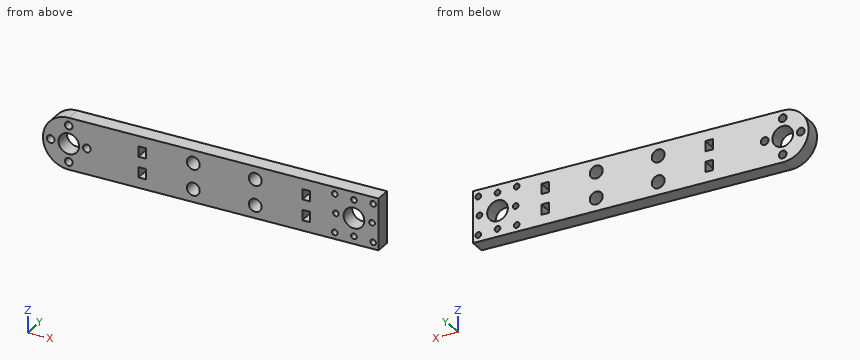
from build123d import *

# Parameters (mm, degrees)
EXTRUDE_1_DEPTH     = 6
SKETCH_2_R          = 1.5
SKETCH_2_R_2        = 4
CUT_EXTRUDE_1_DEPTH = 10
SKETCH_3_W          = 3
SKETCH_3_H          = 4
CUT_EXTRUDE_2_DEPTH = 10
SKETCH_4_R          = 4
SKETCH_4_R_2        = 1.1
SKETCH_4_W          = 3
SKETCH_4_H          = 4
CUT_EXTRUDE_4_DEPTH = 10
SKETCH_5_R          = 2.5
CUT_EXTRUDE_5_DEPTH = 10


with BuildPart() as part:
    # 草图1 → 凸台-拉伸1 (new body)
    with BuildSketch(Plane(origin=(0, 0, 0), x_dir=(1, 0, 0), z_dir=(0, 1, 0))):
        with BuildLine():
            Line((-41.199983302, 20), (78.800016698, 20))
            Line((78.800016698, 20), (78.800016698, 0))
            Line((78.800016698, 0), (-41.199983302, 0))
            ThreePointArc((-41.199983302, 0), (-51.199983302, 10), (-41.199983302, 20))
        make_face()
    extrude(amount=EXTRUDE_1_DEPTH)

    # 草图2 → 切除-拉伸1 (cut)
    with BuildSketch(Plane(origin=(0, 6, 0), x_dir=(1, 0, 0), z_dir=(0, 1, 0))):
        with Locations(Location((-48.199983302, 10, 0), (0, 0, 270))):
            Circle(SKETCH_2_R)
        with BuildLine():
            ThreePointArc((-39.699983302, 17), (-40.13932313, 18.060660172), (-41.199983302, 18.5))
            Line((-41.199983302, 18.5), (-41.199983302, 17))
            Line((-41.199983302, 17), (-41.199983302, 15.5))
            ThreePointArc((-41.199983302, 15.5), (-40.13932313, 15.939339828), (-39.699983302, 17))
        make_face()
        with BuildLine():
            Line((-41.199983302, 17), (-41.199983302, 18.5))
            ThreePointArc((-41.199983302, 18.5), (-42.699983302, 17), (-41.199983302, 15.5))
            Line((-41.199983302, 15.5), (-41.199983302, 17))
        make_face()
        with Locations(Location((-34.199983302, 10, 0), (0, 0, 270))):
            Circle(SKETCH_2_R)
        with BuildLine():
            ThreePointArc((-39.699983302, 3), (-40.13932313, 4.060660172), (-41.199983302, 4.5))
            Line((-41.199983302, 4.5), (-41.199983302, 3))
            Line((-41.199983302, 3), (-41.199983302, 1.5))
            ThreePointArc((-41.199983302, 1.5), (-40.13932313, 1.939339828), (-39.699983302, 3))
        make_face()
        with BuildLine():
            Line((-41.199983302, 3), (-41.199983302, 4.5))
            ThreePointArc((-41.199983302, 4.5), (-42.699983302, 3), (-41.199983302, 1.5))
            Line((-41.199983302, 1.5), (-41.199983302, 3))
        make_face()
        with Locations(Location((-41.199983302, 10, 0), (0, 0, 270))):
            Circle(SKETCH_2_R_2)
    extrude(amount=-CUT_EXTRUDE_1_DEPTH, mode=Mode.SUBTRACT)

    # 草图3 → 切除-拉伸2 (cut)
    with BuildSketch(Plane(origin=(0, 6, 0), x_dir=(1, 0, 0), z_dir=(0, 1, 0))):
        with Locations((-12.699983302, 14)):
            Rectangle(SKETCH_3_W, SKETCH_3_H)
        with Locations((-12.699983302, 6)):
            Rectangle(SKETCH_3_W, SKETCH_3_H)
    extrude(amount=-CUT_EXTRUDE_2_DEPTH, mode=Mode.SUBTRACT)

    # 草图4 → 切除-拉伸4 (cut)
    with BuildSketch(Plane(origin=(0, 6, 0), x_dir=(1, 0, 0), z_dir=(0, 1, 0))):
        with Locations(Location((69.300016698, 10, 0), (0, 0, 270))):
            Circle(SKETCH_4_R)
        with Locations(Location((76.7246379, 17.424621202, 0), (0, 0, 270))):
            Circle(SKETCH_4_R_2)
        with Locations(Location((62.300016698, 10, 0), (0, 0, 270))):
            Circle(SKETCH_4_R_2)
        with Locations((50.800016698, 6)):
            Rectangle(SKETCH_4_W, SKETCH_4_H)
        with Locations((50.800016698, 14)):
            Rectangle(SKETCH_4_W, SKETCH_4_H)
        with Locations(Location((76.7246379, 2.575378798, 0), (0, 0, 270))):
            Circle(SKETCH_4_R_2)
        with Locations(Location((61.875395496, 2.575378798, 0), (0, 0, 270))):
            Circle(SKETCH_4_R_2)
        with Locations(Location((61.875395496, 17.424621202, 0), (0, 0, 270))):
            Circle(SKETCH_4_R_2)
        with Locations(Location((69.300016698, 17, 0), (0, 0, 270))):
            Circle(SKETCH_4_R_2)
        with Locations(Location((76.300016698, 10, 0), (0, 0, 270))):
            Circle(SKETCH_4_R_2)
        with Locations(Location((69.300016698, 3, 0), (0, 0, 270))):
            Circle(SKETCH_4_R_2)
    extrude(amount=-CUT_EXTRUDE_4_DEPTH, mode=Mode.SUBTRACT)

    # 草图5 → 切除-拉伸5 (cut)
    with BuildSketch(Plane(origin=(0, 6, 0), x_dir=(1, 0, 0), z_dir=(0, 1, 0))):
        with Locations(Location((31.050016698, 15, 0), (0, 0, 270))):
            Circle(SKETCH_5_R)
        with Locations(Location((31.050016698, 5, 0), (0, 0, 270))):
            Circle(SKETCH_5_R)
        with Locations(Location((7.050016698, 15, 0), (0, 0, 270))):
            Circle(SKETCH_5_R)
        with Locations(Location((7.050016698, 5, 0), (0, 0, 270))):
            Circle(SKETCH_5_R)
    extrude(amount=-CUT_EXTRUDE_5_DEPTH, mode=Mode.SUBTRACT)


solid = part.part
Verification items for the finished model (mm, model axes). Coordinates: 2 decimals unless noted, no trailing zeros. Order: outer loops, then holes, each group sorted by start corner. A loop starts at its lowest first (then second) coordinate and runs counter-clockwise, first axis right, second up.
1. Go/stop test with flat-tipped pins: pin 1 Ø6 at (x, z) = (7.05, -15) entering from -Y; pin 2 Ø2 at (y, z) = (4, -14.5) entering from -X. Record where each tip stops, or that it passes through.
Results found:
pin 1: stops at y = 0
pin 2: stops at x = -50.57
2. Sectioned sample at B-B, the plane y = 4.3. Give the number of separate pieces and of enclosed holes in the cut face, and give its area (3 significant figures).
Results found:
separate pieces: 1
enclosed holes: 22
area: 2,270 mm2
3. Sectioned sample at A-A, the plane z = -10. Record the cut outline in (x, y).
Results found:
outline: (-51.2, 0) - (-49.7, 0) - (-49.7, 6) - (-51.2, 6) - close; (-46.7, 0) - (-45.2, 0) - (-45.2, 6) - (-46.7, 6) - close; (-37.2, 0) - (-35.7, 0) - (-35.7, 6) - (-37.2, 6) - close; (-32.7, 0) - (61.2, 0) - (61.2, 6) - (-32.7, 6) - close; (63.4, 0) - (65.3, 0) - (65.3, 6) - (63.4, 6) - close; (73.3, 0) - (75.2, 0) - (75.2, 6) - (73.3, 6) - close; (77.4, 0) - (78.8, 0) - (78.8, 6) - (77.4, 6) - close
4. Scan lines: line 1 (Z direction, x = 7, y = 0.9); line 2 (Z direction, x = 51, y = 5.65); line 3 (Z direction, x = -37.5, y = 2.9). Record each from-to range of solid material in increasing order.
Results found:
line 1: z = -20 to -17.5, -12.5 to -7.5, -2.5 to 0
line 2: z = -20 to -16, -12 to -8, -4 to 0
line 3: z = -20 to -11.52, -8.48 to 0
